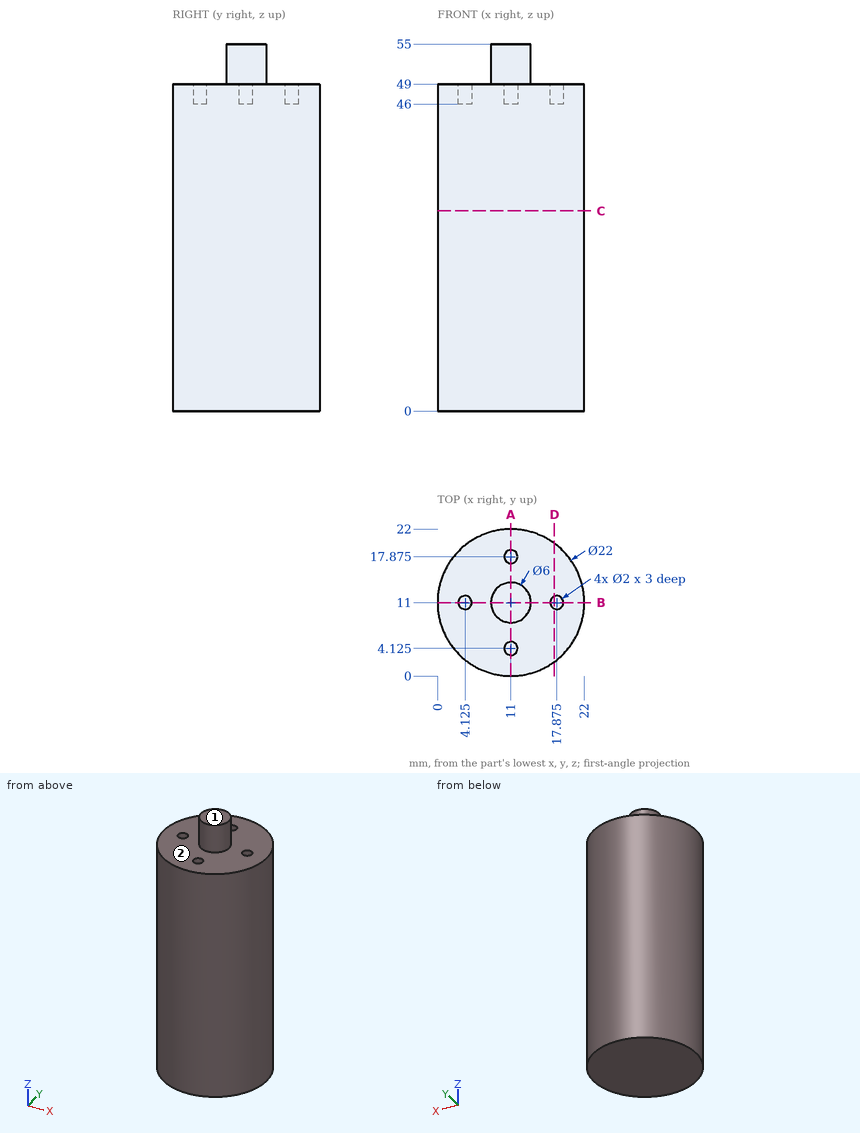
The figure shows three views and two pictorial views of one solid part (mm, origin at its lowest corner). Answer the questions. A direction names the side the tool comes from. Round coordinates to 2 decimals unless told otherwise and drop trailing zeros. Write each loop counter-clockwise with the first axis right and the second up, starting at its lowest first coordinate (ties: lowest second). Pieces come first, ordered by that corner, then holes. Notation, with made-up numbers: M 55.25,-11.5 L 91.25,-11.5 A28 ccw 91.25,27.5 Z; hole C -14.5,53.5 d5. An arc over 180 degrees is marked long. Use a Markdown table: item, result.
1) Which of the six approach directions +Z, -Z, +X, -X, +Y, -Y give full straight-line access (tool end or side, diameter ignored) to the marked faces 1 and 2?
Taken from the geometry:
| item | result |
|---|---|
| face 1 | +Z, +X, -X, +Y, -Y |
| face 2 | +Z |
2) The part is cut by section A-A on x = 11. Give the vertices of the cut face in (y, z) (3 decimals).
Taken from the geometry:
| item | result |
|---|---|
| outline | M 0,0 L 22,0 L 22,49 L 18.875,49 L 18.875,46 L 16.875,46 L 16.875,49 L 14,49 L 14,55 L 8,55 L 8,49 L 5.125,49 L 5.125,46 L 3.125,46 L 3.125,49 L 0,49 Z |
3) The part is cut by section D-D on x = 17.5. Give the vertices of the cut face in (y, z).
Taken from the geometry:
| item | result |
|---|---|
| outline | M 2.13,0 L 19.87,0 L 19.87,49 L 11.93,49 L 11.93,46 L 10.07,46 L 10.07,49 L 2.13,49 Z |
4) The part is cut by section C-C on z = 30. Give the vertices of the cut face in (x, y).
Taken from the geometry:
| item | result |
|---|---|
| outline | C 11,11 d22 |
5) Flat-ended cylindrical pins translate along their axes: pin 1 (1 mm diameter, centred on x = 11, y = 4.5, fed in from +Z); pin 2 (3 mm diameter, centred on y = 8.5, z = 39, fed in from -X); pin 3 (3 mm diameter, centred on x = 11, y = 17.875, fed in from +Z). Find the tip coordinate at first contact, or state that the pin passes through.
Taken from the geometry:
| item | result |
|---|---|
| pin 1 | stops at z = 46 |
| pin 2 | stops at x = 0.05 |
| pin 3 | stops at z = 49 |
6) Consider line 1 (Y direction, x = 11, z = 47.7) (3 decimals); line 2 (Z direction, x = 4.25, y = 10.75); line 3 (Z direction, x = 12.5, y = 6.25). Determine where each line is inside the solid, lowest interval first. Write a range as [from, to].
Taken from the geometry:
| item | result |
|---|---|
| line 1 | y = [0, 3.125], [5.125, 16.875], [18.875, 22] |
| line 2 | z = [0, 46] |
| line 3 | z = [0, 49] |
